```python
from build123d import *

# Parameters (mm, degrees)
SKETCH1_W          = 76.2
SKETCH1_H          = 6.985
SKETCH1_W_2        = 15.24
SKETCH1_H_2        = 6.35
SKETCH2_R          = 5.565762573
CUT_EXTRUDE1_DEPTH = 106.68


with BuildPart() as part:
    # Sketch1 → Revolve1 (revolve)
    with BuildSketch(Plane.XY, mode=Mode.PRIVATE) as revolve1_sk:
        with Locations((38.1, 3.4925)):
            Rectangle(SKETCH1_W, SKETCH1_H)
        with Locations((83.82, 3.175)):
            Rectangle(SKETCH1_W_2, SKETCH1_H_2)
        with Locations((-7.62, 3.175)):
            Rectangle(SKETCH1_W_2, SKETCH1_H_2)
    revolve(revolve1_sk.sketch.rotate(Axis((-92.340325691, 0, 0), (1, 0, 0)), 90), axis=Axis((-92.340325691, 0, 0), (1, 0, 0)))

    # Sketch2 → Cut-Extrude1 (cut)
    with BuildSketch(Plane(origin=(91.44, 0, 0), x_dir=(0, 0, -1), z_dir=(1, 0, 0))):
        Circle(SKETCH2_R)
    extrude(amount=-CUT_EXTRUDE1_DEPTH, mode=Mode.SUBTRACT)


solid = part.part
```
Here's how the part is built. I have some questions about the finished solid (model axes, mm). A direction names the side the tool comes from. Round coordinates to 2 decimals unless told otherwise and drop trailing zeros. Loops run counter-clockwise (first coordinate to the right, second up) from the corner with the lowest first, then second, coordinate; pieces in that order, holes last. Notation, with made-up numbers: (88.5, -6) -> (143.5, -6) arc R36 cw to (143.5, 31) -> close; hole circle Ø7 at (75, -8.75). An arc over 180 degrees is marked (long way). Answer as CSV lines item,"result". Start each with the question number.
1. For faces 1 (the face through (0, 6, -3)), 2 (the face through (76.2, 6, -3)), 3 (the face through (38.633, -6.926, -0.909)), which set-ups out of +Z, -Z, +X, -X, +Y, -Y let a thin tool reach every point of the face, with its end or its side?
2. Imagine slicing it at A-A on y = 0. Write out the boundary of the cut face in (x, z) (3 decimals), plus the area to 3 significant figures.
3. Imagine slicing it at C-C on x = 9. Write out the boundary of the cut face in (y, z) (3 decimals), plus the area to 3 significant figures.
4. I'm going to push flat-ended pins straight in: P1, Ø1, axis at x = 68.5, z = 1, coming from the +Y side; P2, Ø1.5, axis at x = 49, y = -2, coming from the +Z side; P3, Ø4, axis at x = -3.5, y = 4, coming from the +Z side. Where does each tip first touch, or does it pass through?
5. If we mould it in two halves opening along Z, with no side actions, what happens to faces 4 (the face through (91.44, 6, 0)), 5 (the face through (38.847, -5.433, 1.207)), 6 (the face through (-7.51, 3.86, -5.04))? For each: pulls with the +Z half, pulls with the -Z half, needs draft (parallel to the pull), parting line crosses it, or undercut.
6. I need wall thicknesses on probe 1 along Y at (x, z) = (6, 0) (3 decimals); probe 2 along Z at (x, y) = (1, -2.5); probe 3 along Y at (x, z) = (59.5, 3.25). Which ranges of each line are inside material? Lowest first, please. Write a range as from..to.
Solution:
1,face 1,"-X"
1,face 2,"+X"
1,face 3,"+X, -X"
2,outline,"(-15.24, -6.35) -> (0, -6.35) -> (0, -6.985) -> (76.2, -6.985) -> (76.2, -6.35) -> (91.44, -6.35) -> (91.44, -5.566) -> (-15.24, -5.566) -> close; (-15.24, 5.566) -> (91.44, 5.566) -> (91.44, 6.35) -> (76.2, 6.35) -> (76.2, 6.985) -> (0, 6.985) -> (0, 6.35) -> (-15.24, 6.35) -> close"
2,area,"264 mm²"
3,outline,"circle Ø13.97 at (0, 0); hole circle Ø11.132 at (0, 0)"
3,area,"56.0 mm²"
4,P1,"y = 6.97"
4,P2,"z = 6.87"
4,P3,"z = 6.03"
5,face 4,"needs draft"
5,face 5,"undercut"
5,face 6,"parting line crosses it"
6,probe 1,"-6.985..-5.566, 5.566..6.985"
6,probe 2,"-6.52..-4.97, 4.97..6.52"
6,probe 3,"-6.18..-4.52, 4.52..6.18"
